```python
from build123d import *

# Parameters (mm, degrees)
SKETCH_1_R          = 26.15
EXTRUDE_1_DEPTH     = 1
SKETCH_2_R          = 24.15
EXTRUDE_2_DEPTH     = 1
SKETCH_3_R          = 1.5
CUT_EXTRUDE_1_DEPTH = 3


with BuildPart() as part:
    # Эскиз1 → Бобышка-Вытянуть1 (new body)
    with BuildSketch(Plane(origin=(0, 0, 0), x_dir=(1, 0, 0), z_dir=(0, 1, 0))):
        Circle(SKETCH_1_R)
    extrude(amount=EXTRUDE_1_DEPTH)

    # Эскиз2 → Бобышка-Вытянуть2 (add)
    with BuildSketch(Plane(origin=(0, 1, 0), x_dir=(1, 0, 0), z_dir=(0, 1, 0))):
        Circle(SKETCH_2_R)
    extrude(amount=EXTRUDE_2_DEPTH)

    # Эскиз3 → Вырез-Вытянуть1 (cut, through all)
    with BuildSketch(Plane(origin=(0, 2, 0), x_dir=(1, 0, 0), z_dir=(0, 1, 0))):
        Circle(SKETCH_3_R)
        with Locations((5, 0)):
            Circle(SKETCH_3_R)
        with Locations((10, 0)):
            Circle(SKETCH_3_R)
        with Locations((15, 0)):
            Circle(SKETCH_3_R)
        with Locations((20, 0)):
            Circle(SKETCH_3_R)
        with Locations((2.5, -4.330127019)):
            Circle(SKETCH_3_R)
        with Locations((5, -8.660254038)):
            Circle(SKETCH_3_R)
        with Locations((7.5, -12.990381057)):
            Circle(SKETCH_3_R)
        with Locations((10, -17.320508076)):
            Circle(SKETCH_3_R)
        with Locations((-2.5, -4.330127019)):
            Circle(SKETCH_3_R)
        with Locations((-5, -8.660254038)):
            Circle(SKETCH_3_R)
        with Locations((-7.5, -12.990381057)):
            Circle(SKETCH_3_R)
        with Locations((-10, -17.320508076)):
            Circle(SKETCH_3_R)
        with Locations((-5, 0)):
            Circle(SKETCH_3_R)
        with Locations((-10, 0)):
            Circle(SKETCH_3_R)
        with Locations((-15, 0)):
            Circle(SKETCH_3_R)
        with Locations((-20, 0)):
            Circle(SKETCH_3_R)
        with Locations((-2.5, 4.330127019)):
            Circle(SKETCH_3_R)
        with Locations((-5, 8.660254038)):
            Circle(SKETCH_3_R)
        with Locations((-7.5, 12.990381057)):
            Circle(SKETCH_3_R)
        with Locations((-10, 17.320508076)):
            Circle(SKETCH_3_R)
        with Locations((2.5, 4.330127019)):
            Circle(SKETCH_3_R)
        with Locations((5, 8.660254038)):
            Circle(SKETCH_3_R)
        with Locations((7.5, 12.990381057)):
            Circle(SKETCH_3_R)
        with Locations((10, 17.320508076)):
            Circle(SKETCH_3_R)
        with Locations((8.660254038, -5)):
            Circle(SKETCH_3_R)
        with Locations((12.990381057, -7.5)):
            Circle(SKETCH_3_R)
        with Locations((17.320508076, -10)):
            Circle(SKETCH_3_R)
        with Locations((0, -10)):
            Circle(SKETCH_3_R)
        with Locations((0, -15)):
            Circle(SKETCH_3_R)
        with Locations((0, -20)):
            Circle(SKETCH_3_R)
        with Locations((-8.660254038, -5)):
            Circle(SKETCH_3_R)
        with Locations((-12.990381057, -7.5)):
            Circle(SKETCH_3_R)
        with Locations((-17.320508076, -10)):
            Circle(SKETCH_3_R)
        with Locations((-8.660254038, 5)):
            Circle(SKETCH_3_R)
        with Locations((-12.990381057, 7.5)):
            Circle(SKETCH_3_R)
        with Locations((-17.320508076, 10)):
            Circle(SKETCH_3_R)
        with Locations((0, 10)):
            Circle(SKETCH_3_R)
        with Locations((0, 15)):
            Circle(SKETCH_3_R)
        with Locations((0, 20)):
            Circle(SKETCH_3_R)
        with Locations((8.660254038, 5)):
            Circle(SKETCH_3_R)
        with Locations((12.990381057, 7.5)):
            Circle(SKETCH_3_R)
        with Locations((17.320508076, 10)):
            Circle(SKETCH_3_R)
        with Locations((14.488887394, -3.882285677)):
            Circle(SKETCH_3_R)
        with Locations((19.318516526, -5.176380902)):
            Circle(SKETCH_3_R)
        with Locations((10.606601718, -10.606601718)):
            Circle(SKETCH_3_R)
        with Locations((14.142135624, -14.142135624)):
            Circle(SKETCH_3_R)
        with Locations((3.882285677, -14.488887394)):
            Circle(SKETCH_3_R)
        with Locations((5.176380902, -19.318516526)):
            Circle(SKETCH_3_R)
        with Locations((-3.882285677, -14.488887394)):
            Circle(SKETCH_3_R)
        with Locations((-5.176380902, -19.318516526)):
            Circle(SKETCH_3_R)
        with Locations((-10.606601718, -10.606601718)):
            Circle(SKETCH_3_R)
        with Locations((-14.142135624, -14.142135624)):
            Circle(SKETCH_3_R)
        with Locations((-14.488887394, -3.882285677)):
            Circle(SKETCH_3_R)
        with Locations((-19.318516526, -5.176380902)):
            Circle(SKETCH_3_R)
        with Locations((-14.488887394, 3.882285677)):
            Circle(SKETCH_3_R)
        with Locations((-19.318516526, 5.176380902)):
            Circle(SKETCH_3_R)
        with Locations((-10.606601718, 10.606601718)):
            Circle(SKETCH_3_R)
        with Locations((-14.142135624, 14.142135624)):
            Circle(SKETCH_3_R)
        with Locations((-3.882285677, 14.488887394)):
            Circle(SKETCH_3_R)
        with Locations((-5.176380902, 19.318516526)):
            Circle(SKETCH_3_R)
        with Locations((3.882285677, 14.488887394)):
            Circle(SKETCH_3_R)
        with Locations((5.176380902, 19.318516526)):
            Circle(SKETCH_3_R)
        with Locations((10.606601718, 10.606601718)):
            Circle(SKETCH_3_R)
        with Locations((14.142135624, 14.142135624)):
            Circle(SKETCH_3_R)
        with Locations((14.488887394, 3.882285677)):
            Circle(SKETCH_3_R)
        with Locations((19.318516526, 5.176380902)):
            Circle(SKETCH_3_R)
    extrude(amount=-CUT_EXTRUDE_1_DEPTH, mode=Mode.SUBTRACT)


solid = part.part
```
Verification items for the finished model (mm, model axes). Round coordinates to 2 decimals unless told otherwise and drop trailing zeros. Write each loop counter-clockwise with the first axis right and the second up, starting at its lowest first coordinate (ties: lowest second). Pieces come first, ordered by that corner, then holes. Notation, with made-up numbers: (-13, -21.75) - (14, -21.75) arc R24 cw to (14, -0.75) - close; hole circle Ø10 at (50.25, -15.75). An arc over 180 degrees is marked (long way). Answer as a JSON object with one key per item and string values. Group by question number.
Q1. Thickness scan on line 1 (X direction, y = 0.75, z = 18); line 2 (X direction, y = 1.2, z = -3); line 3 (Z direction, x = -17, y = 0.3). Record the ranges inside material, lowest first.
Q2. Section check A-A, the plane x = -20. Enter the section's corners in (y, z), plus the area to 3 significant figures.
Q3. Mould release check, pull along X, two halves, no side actions. Record for faces 1 (the cylindrical face through (-24.127, 1.493, -1.062)), 2 (the cylindrical face through (-9.8, 1.01, -11.87)), 3 (the flat face through (0, 0, -6)): released by +X, released by -X, zero draft, split by the parting line, or undercut.
Q4. Section check B-B, the plane z = 0. Give the number of separate pieces and of enclosed holes in the cut face, plus the area to 3 significant figures.
Q5. Go/stop test with a flat-tipped pin: pin 1 Ø2.5 at (x, z) = (0, -20) entering from +Y. Record where the tip stops, or that it passes through.
Found:
{
 "1": {"line 1": "x = -18.97 to -11.34, -8.66 to -5.89, -4.46 to 4.46, 5.89 to 8.66, 11.34 to 18.97", "line 2": "x = -23.96 to -15.7, -13.28 to -3.19, -1.81 to 1.81, 3.19 to 13.28, 15.7 to 23.96", "line 3": "z = -19.87 to -11.47, -8.53 to 8.53, 11.47 to 19.87"},
 "2": {"outline": "(0, -16.85) - (1, -16.85) - (1, -13.54) - (2, -13.54) - (2, -6.51) - (0, -6.51) - close; (0, -3.84) - (2, -3.84) - (2, -1.5) - (0, -1.5) - close; (0, 1.5) - (2, 1.5) - (2, 3.84) - (0, 3.84) - close; (0, 6.51) - (2, 6.51) - (2, 13.54) - (1, 13.54) - (1, 16.85) - (0, 16.85) - close", "area": "44.1 mm^2"},
 "3": {"face 1": "split by the parting line", "face 2": "undercut", "face 3": "zero draft"},
 "4": {"separate pieces": "10", "enclosed holes": "0", "area": "46.6 mm^2"},
 "5": {"pin 1": "passes through"}
}
